from build123d import *

# Parameters (mm, degrees)
F1_DEPTH      = 146.05
F2_R          = 3.175
F3_DEPTH      = 19.051
F4_R          = 6.35
F6_DEPTH      = 9.652
F7_R          = 19.05
F8_DEPTH      = 25.4
F8_DEPTH_BACK = 20.6375
F9_R          = 9.525
F10_DEPTH     = 46.0385
F11_W         = 44.45
F11_H         = 50.8
F12_DEPTH     = 9.652
F13_R         = 3.175
F14_DEPTH     = 9.652
F15_W         = 9.652
F15_H         = 6.35
F16_DEPTH     = 50.8
F17_R         = 4.826
F18_R         = 3.048


with BuildPart() as f1:
    # F0 (on Right) → F1 (new body)
    with BuildSketch(Plane.YZ):
        Polygon((0, -25.4), (0, 0), (-42.672, 0), (-42.672, -6.35), (-58.674, -6.35), (-58.674, 0), (-73.152, 0), (-73.152, -12.7), (-12.7, -12.7), (-12.7, -25.4), align=None)
    extrude(amount=F1_DEPTH)

    # F2 (on face) → F3 (cut, through all)
    with BuildSketch(Plane.XY.offset(-6.35)):
        with Locations((107.95, -50.673)):
            Circle(F2_R)
        with Locations((38.1, -50.673)):
            Circle(F2_R)
    extrude(amount=-F3_DEPTH, mode=Mode.SUBTRACT)

    # F4
    f4_edges = [f1.edges().sort_by_distance(p)[0] for p in [
        (73.025, 0, -25.4),
    ]]
    fillet(f4_edges, radius=F4_R)

    # F5 (on face) → F6 (join)
    with BuildSketch(Plane(origin=(0, 0, 0), x_dir=(-1, 0, 0), z_dir=(0, 1, 0))):
        Polygon((-20.2930348437, 35.148567389), (-34.798, 47.498), (-50.2252331933, 58.674), (-111.237689279, 93.899557945), (-136.398, 0), (0, 0), align=None)
    extrude(amount=-F6_DEPTH)

    # F7 (on face) → F8 (join, two sides)
    with BuildSketch(Plane(origin=(0, 0, 0), x_dir=(-1, 0, 0), z_dir=(0, 1, 0))) as f8_sk:
        with Locations((-34.798, 47.498)):
            Circle(F7_R)
    extrude(amount=-F8_DEPTH)
    extrude(f8_sk.sketch, amount=F8_DEPTH_BACK)

    # F9 (on face) → F10 (cut, through all)
    with BuildSketch(Plane.XZ.offset(25.4)):
        with Locations((34.798, 47.498)):
            Circle(F9_R)
    extrude(amount=-F10_DEPTH, mode=Mode.SUBTRACT)

    # F11 (on face) → F12 (join)
    with BuildSketch(Plane(origin=(127.2610665127, 0, 34.0995), x_dir=(0, 1, 0), z_dir=(0.9659258263, 0, 0.2588190451))):
        with Locations((-4.826, 39.534108053)):
            Rectangle(F11_W, F11_H)
    extrude(amount=F12_DEPTH)

    # F13 (on face) → F14 (cut)
    with BuildSketch(Plane(origin=(136.584182588, 0, 36.5976214233), x_dir=(0, 1, 0), z_dir=(0.9659258263, 0, 0.2588190451))):
        with Locations((-17.526, 55.409108053)):
            Circle(F13_R)
        with Locations((7.874, 55.409108053)):
            Circle(F13_R)
        with Locations((7.874, 23.659108053)):
            Circle(F13_R)
        with Locations((-17.526, 23.659108053)):
            Circle(F13_R)
    extrude(amount=-F14_DEPTH, mode=Mode.SUBTRACT)

    # F15 (on face) → F16 (join)
    with BuildSketch(Plane(origin=(-16.8061838409, 0, 62.7215319755), x_dir=(0.9659258263, 0, 0.2588190451), z_dir=(-0.2588190451, 0, 0.9659258263))):
        with Locations((146.2283508542, -4.826)):
            Rectangle(F15_W, F15_H)
    extrude(amount=-F16_DEPTH)

    # F17
    f17_edges = [f1.edges().sort_by_distance(p)[0] for p in [
        (115.116441, -27.051, 98.070093),
        (115.116441, 17.399, 98.070093),
        (128.264448, -27.051, 49.001061),
        (128.264448, 17.399, 49.001061),
    ]]
    fillet(f17_edges, radius=F17_R)

    # F18
    f18_edges = [f1.edges().sort_by_distance(p)[0] for p in [
        (46.569752, 0, 32.520405),
        (46.569752, -9.652, 32.520405),
        (68.199, -9.652, 0),
    ]]
    fillet(f18_edges, radius=F18_R)


solid = f1.part
For this review, take the finished solid that the model builds, in its own axes (mm). A direction names the side the tool comes from. Give positions to 0.01 mm unless a question says otherwise; leave off trailing zeros. Loops run counter-clockwise (first coordinate to the right, second up) from the corner with the lowest first, then second, coordinate; pieces in that order, holes last.
Item 1: Tool access review of faces 4 (the flat face through (122, -27.051, 73)), 5 (the flat face through (72, -58.674, -3)), 6 (the flat face through (129.91, -4.85, 24.21)), 7 (the flat face through (116.937, -10.076, 72.63)), 8 (the flat face through (72, -12.7, -19)): name each direction out of +Z, -Z, +X, -X, +Y, -Y from which nothing blocks a thin tool from reaching the whole face with its end or side.
Item 2: For line 1 along Y through (x, z) = (107.95, -8); line 2 along Z through (x, y) = (84, -27); line 3 along Y through (x, z) = (44, 26), list the stretches that pass through material, from the lowest coordinate up.
Item 3: Take a section at D-D, the plane x = 38.1. Give the number of separate pieces and of enclosed holes in the cut face, and give its area (3 significant figures).
Item 4: Take a section at B-B, the plane z = 73.5. State the section outline as (x, y) points, and give its area (3 significant figures).
Item 5: Draft analysis for pull direction Z (two halves, no side actions). For faces 1 (the cylindrical face through (126.179, 10.807, 57.044)), 2 (the cylindrical face through (37.687, -47.525, -9.481)), 3 (the cylindrical face through (74.05, -1.81, -23.49)), state which applies: +Z half, -Z half, draft (parallel to the pull), parting line (faces both ways), or undercut.
Item 6: Take a section at C-C, the plane x = 83.5. State the section outline as (y, z) points, and give its area (3 significant figures).
Item 7: Insertion check: pin 1 (6 mm diameter, centred on x = 124, z = 63.5, fed in from -Y); pin 2 (7.5 mm diameter, centred on x = 107.95, y = -50.673, fed in from +Z); pin 3 (6 mm diameter, centred on x = 100.5, y = -31, fed in from +Z). Each pin has a flat end and moves straight along its axis. Give the tip position at first contact, or say it passes through.
Item 8: Take a section at A-A, the plane x = 107.95. State the section outline as (y, z) points, and give its area (3 significant figures).
Calculated:
1. face 4: +Z, +X, -X, -Y
1. face 5: +Z, +X, -X
1. face 6: +X, +Y, -Y
1. face 7: none
1. face 8: -Z, +X, -X, -Y
2. line 1: y = -73.15 to -53.85, -47.5 to 0
2. line 2: z = -12.7 to 0
2. line 3: y = -9.65 to 0
3. separate pieces: 3
3. enclosed holes: 0
3. area: 2,130 mm2
4. outline: (75.9, -9.65) - (116.7, -9.65) - (116.7, -27.05) - (126.7, -27.05) - (126.7, -8) - (136.69, -8) - (136.69, -1.65) - (126.7, -1.65) - (126.7, 17.4) - (116.7, 17.4) - (116.7, 0) - (75.9, 0) - close
4. area: 901 mm2
5. face 1: undercut
5. face 2: draft
5. face 3: -Z half
6. outline: (-73.15, -12.7) - (-12.7, -12.7) - (-12.7, -25.4) - (-6.35, -25.4) arc R6.35 ccw to (0, -19.05) - (0, 77.89) - (-9.65, 77.89) - (-9.65, 3.05) arc R3.05 cw to (-12.7, 0) - (-42.67, 0) - (-42.67, -6.35) - (-58.67, -6.35) - (-58.67, 0) - (-73.15, 0) - close
6. area: 1,730 mm2
7. pin 1: stops at y = -27.05
7. pin 2: stops at z = -6.35
7. pin 3: stops at z = 0
8. outline: (-73.15, -12.7) - (-53.85, -12.7) - (-53.85, -6.35) - (-58.67, -6.35) - (-58.67, 0) - (-73.15, 0) - close; (-47.5, -12.7) - (-12.7, -12.7) - (-12.7, -25.4) - (-6.35, -25.4) arc R6.35 ccw to (0, -19.05) - (0, 92) - (-9.65, 92) - (-9.65, 3.05) arc R3.05 cw to (-12.7, 0) - (-42.67, 0) - (-42.67, -6.35) - (-47.5, -6.35) - close
8. area: 1,830 mm2
